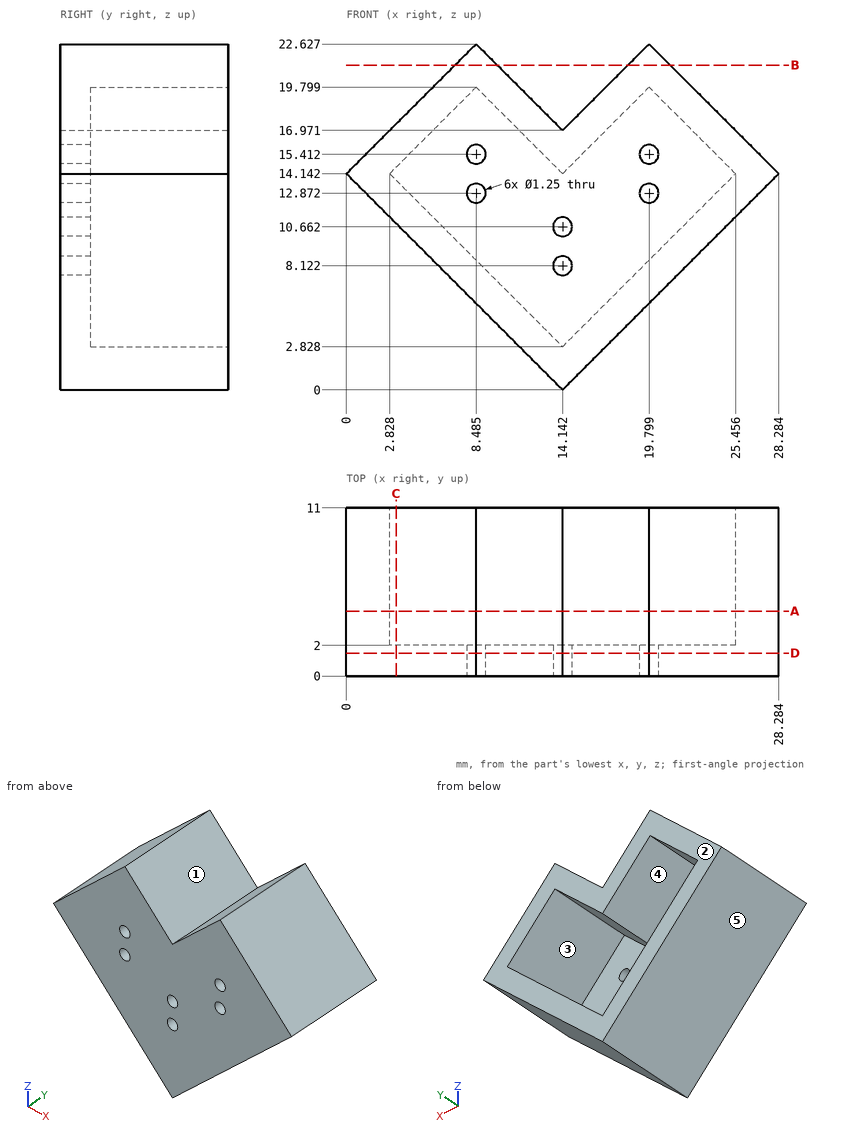
Source: three-view drawing plus pictorial views. Frame: mm from the lowest corner of the part. A direction names the side the tool comes from. Coordinates: 2 decimals unless noted, no trailing zeros. Loops run counter-clockwise (first coordinate to the right, second up) from the corner with the lowest first, then second, coordinate; pieces in that order, holes last. Notation, with made-up numbers: (-0.5, -6) - (56.5, -6) arc R31 ccw to (56.5, 32) - close; hole circle Ø7 at (-22, 38.5). An arc over 180 degrees is marked (long way). Answer in a Markdown table with one row per item. Add a question column.
Item 1: Section query A-A on y = 4.25. Return the cut outline in (x, z) (1 decimal).
Item 2: Mould query, pull axis Z, two halves, no side actions, for the marked faces 1, 2 and 3. Classes: released by +Z, released by -Z, zero draft, split by the parting line, or undercut.
Item 3: Line query: line 1 along X through (y, z) = (10.25, 16) (1 decimal); line 2 along X through (y, z) = (9.5, 15.5) (1 decimal); line 3 along X through (y, z) = (6.75, 18) (1 decimal). Output: solid intervals per line, ascending. Write a range as [from, to].
Item 4: Section query D-D on y = 1.5. State how many separate pieces and enclosed holes the cut face has, then the cut area to 3 significant figures.
Item 5: Contact query for flat-ended pins moving along their axis: P1, Ø6, axis at x = 4, y = 10, coming from the -Z side; P2, Ø1.1, axis at x = 14.14, z = 10.66, coming from the -Y side; P3, Ø3, axis at y = 6, z = 17, coming from the -X side; P4, Ø1.4, axis at x = 19.8, z = 12.87, coming from the +Y side. Output: stop coordinate, or through.
Item 6: Section query B-B on z = 21.25. Return the cut outline in (x, y).
Item 7: Section query C-C on x = 3.25. Return the cut outline in (y, z).
Item 8: Access query for the marked faces 4 and 5. Directions: +Z, -Z, +X, -X, +Y, -Y. A direction counts if a zero-diameter tool reaches every point of the face in a straight line with its end or side. Return the directions, or none.
Recorded:
| question | item | result |
|---|---|---|
| 1 | outline | (0, 14.1) - (14.1, 0) - (28.3, 14.1) - (19.8, 22.6) - (14.1, 17) - (8.5, 22.6) - close; hole (2.8, 14.1) - (14.1, 2.8) - (25.5, 14.1) - (19.8, 19.8) - (14.1, 14.1) - (8.5, 19.8) - close |
| 2 | face 1 | released by +Z |
| 2 | face 2 | zero draft |
| 2 | face 3 | undercut |
| 3 | line 1 | [1.9, 4.7], [12.3, 16], [23.6, 26.4] |
| 3 | line 2 | [1.4, 4.2], [12.8, 15.5], [24.1, 26.9] |
| 3 | line 3 | [3.9, 6.7], [10.3, 13.1], [15.2, 18], [21.6, 24.4] |
| 4 | separate pieces | 1 |
| 4 | enclosed holes | 6 |
| 4 | area | 329 mm^2 |
| 5 | P1 | z = 7.14 |
| 5 | P2 | through |
| 5 | P3 | x = 1.36 |
| 5 | P4 | y = 2 |
| 6 | outline | (7.11, 0) - (9.86, 0) - (9.86, 11) - (7.11, 11) - close; (18.42, 0) - (21.18, 0) - (21.18, 11) - (18.42, 11) - close |
| 7 | outline | (0, 10.89) - (11, 10.89) - (11, 13.72) - (2, 13.72) - (2, 14.56) - (11, 14.56) - (11, 17.39) - (0, 17.39) - close |
| 8 | face 4 | +Y |
| 8 | face 5 | -Z, -X, +Y, -Y |
